Check sheet for the drawn part. Datum: minimum x, y, z corner. Units: mm. A direction names the side the tool comes from. Round coordinates to 2 decimals unless told otherwise and drop trailing zeros. Loops run counter-clockwise (first coordinate to the right, second up) from the corner with the lowest first, then second, coordinate; pieces in that order, holes last.
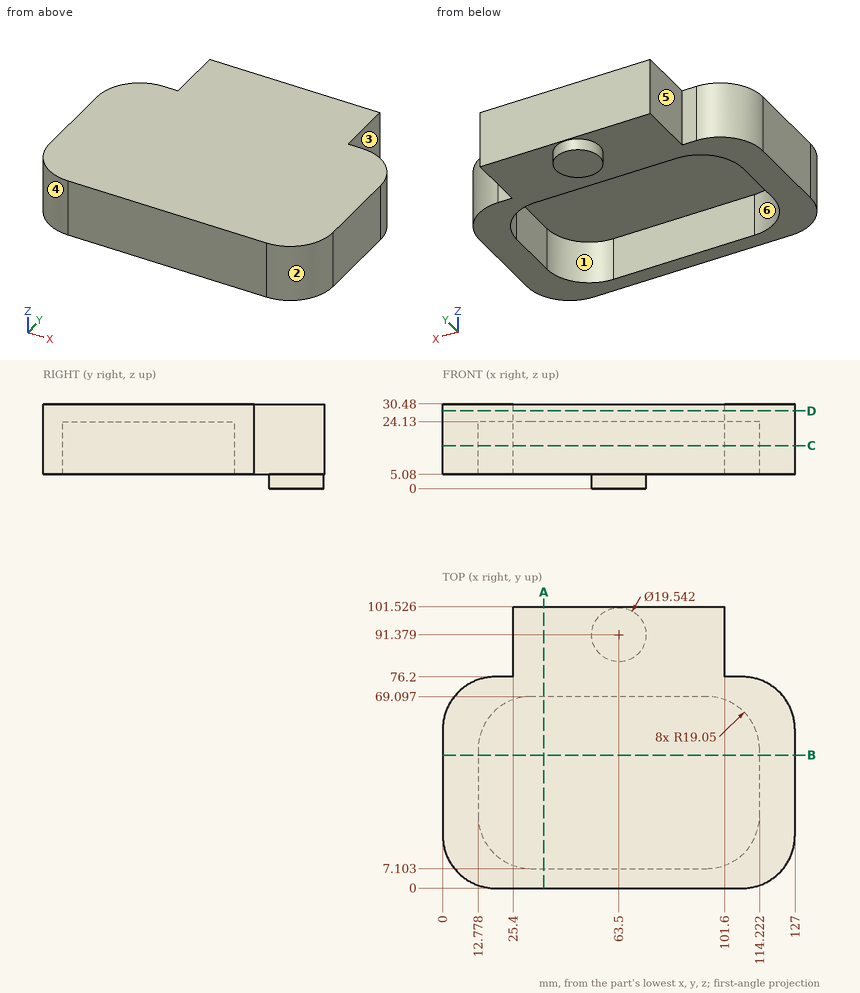
1) Access from +Z, -Z, +X, -X, +Y, -Y to the whole of each face (thin tool, end or side, straight path). Record for the marked faces 1, 2 and 3.
Report:
face 1: -Z
face 2: +Z, -Z, +X, -Y
face 3: +Z, -Z, +X, +Y
2) Sectioned sample at C-C, the plane z = 15.5. Record the cut outline in (x, y).
Report:
outline: (0, 19.05) arc R19.05 ccw to (19.05, 0) - (107.95, 0) arc R19.05 ccw to (127, 19.05) - (127, 57.15) arc R19.05 ccw to (107.95, 76.2) - (101.6, 76.2) - (101.6, 101.53) - (25.4, 101.53) - (25.4, 76.2) - (19.05, 76.2) arc R19.05 ccw to (0, 57.15) - close; hole (12.78, 26.15) arc R19.05 ccw to (31.83, 7.1) - (95.17, 7.1) arc R19.05 ccw to (114.22, 26.15) - (114.22, 50.05) arc R19.05 ccw to (95.17, 69.1) - (31.83, 69.1) arc R19.05 ccw to (12.78, 50.05) - close
3) Mould release check, pull along Y, two halves, no side actions. Record for the marked faces 4, 5 and 6: +Y half, -Y half, draft (parallel to the pull), parting line (faces both ways), or undercut.
Report:
face 4: -Y half
face 5: draft
face 6: undercut
4) Sectioned sample at D-D, the plane z = 28. Record the cut outline in (x, y).
Report:
outline: (0, 19.05) arc R19.05 ccw to (19.05, 0) - (107.95, 0) arc R19.05 ccw to (127, 19.05) - (127, 57.15) arc R19.05 ccw to (107.95, 76.2) - (101.6, 76.2) - (101.6, 101.53) - (25.4, 101.53) - (25.4, 76.2) - (19.05, 76.2) arc R19.05 ccw to (0, 57.15) - close
5) Sectioned sample at A-A, the plane x = 36.5. Record the cut outline in (y, z), then the cut area to 3 significant figures.
Report:
outline: (0, 5.08) - (7.1, 5.08) - (7.1, 24.13) - (69.1, 24.13) - (69.1, 5.08) - (101.53, 5.08) - (101.53, 30.48) - (0, 30.48) - close
area: 1,400 mm2
6) Gauge pin test, flat ends, axial feed: pin 1 (4 mm diameter, centred on x = 104.5, z = 4, fed in from +Y); pin 2 (2 mm diameter, centred on x = 46, z = 4.5, fed in from +Y); pin 3 (18.5 mm diameter, centred on x = 55, y = 48.5, fed in from -Z); pin 4 (7.5 mm diameter, centred on y = 94.5, z = 22, fed in from +X). Record the tip position at first contact, or that the pin passes through.
Report:
pin 1: stops at y = 76.2
pin 2: stops at y = 101.53
pin 3: stops at z = 24.13
pin 4: stops at x = 101.6
7) Scan lines: line 1 along Y through (x, z) = (50, 12.5); line 2 along Z through (x, y) = (27.5, 45.5); line 3 along X through (y, z) = (36, 16). Record each from-to range of solid material in increasing order.
Report:
line 1: y = 0 to 7.1, 69.1 to 101.53
line 2: z = 24.13 to 30.48
line 3: x = 0 to 12.78, 114.22 to 127
8) Sectioned sample at B-B, the plane y = 48. Record the cut outline in (x, z).
Report:
outline: (0, 5.08) - (12.78, 5.08) - (12.78, 24.13) - (114.22, 24.13) - (114.22, 5.08) - (127, 5.08) - (127, 30.48) - (0, 30.48) - close
